Can you work these out from the model? Positions are in its coordinate system, mm. A direction names the side the tool comes from. Give positions to 0.01 mm unless a question says otherwise; leave off trailing zeros. Order: outer loops, then holes, each group sorted by start corner. A loop starts at its lowest first (then second) coordinate and runs counter-clockwise, first axis right, second up. Notation, with made-up numbers: M 87,68.5 L 137,68.5 A7 ccw 137,74.5 Z; hole C 83.25,56 d5. An arc over 180 degrees is marked long. Answer as a JSON object with one key per item and string values.
Autodesk Fusion 360 part; units mm, degrees
sketch "Sketch1" plane through (0, 0, 0) normal (0, 1, 0) x (1, 0, 0)
  line L0 (13.25, -10.25) -> (-13.25, -10.25)
  line L1 (-13.25, -10.25) -> (-13.25, 10.25)
  line L2 (-13.25, 10.25) -> (13.25, 10.25)
  line L3 (13.25, 10.25) -> (13.25, -10.25)
  line L4 (13.25, -10.25) -> (-13.25, 10.25) construction
  line L5 (-13.25, -10.25) -> (13.25, 10.25) construction
  line L6 (-13.25, 10.25) -> (-17.65, 10.25)
  line L7 (-17.65, 10.25) -> (-17.65, 0.25)
  line L8 (-17.65, 0.25) -> (-13.25, 0.25)
  dimension "d1" = 26.5
  dimension "d2" = 20.5
  dimension "d3" = 10
  dimension "d4" = 4.4
extrude "Extrude1" add sketch "Sketch1" along normal blind 1.85
sketch "Sketch2" plane through (0, 1.85, 0) normal (0, 1, 0) x (-1, 0, 0)
  line L0 (-13.25, -10.25) -> (17.65, -10.25)
  line L1 (17.65, -10.25) -> (17.65, -0.25)
  line L2 (17.65, -0.25) -> (13.25, -0.25)
  line L3 (13.25, -0.25) -> (13.25, 10.25)
  line L4 (13.25, 10.25) -> (-13.25, 10.25)
  line L5 (-13.25, 10.25) -> (-13.25, -10.25)
  line L6 (-11, -10.25) -> (-3.4, -10.25)
  line L7 (-3.4, -10.25) -> (-3.4, -5.55)
  line L8 (-3.4, -5.55) -> (-11, -5.55)
  line L9 (-11, -5.55) -> (-11, -10.25)
  dimension "d7" = 7.6
  dimension "d8" = 4.7
  dimension "d9" = 2.25
extrude "Extrude2" add sketch "Sketch2" along normal blind 3.2 contours L0 L6 L7 L8 L9
sketch "Sketch3" plane through (0, 0, 0) normal (0, -1, 0) x (1, 0, 0)
  line L0 (-17.65, -10.25) -> (13.25, -10.25)
  line L1 (13.25, -10.25) -> (13.25, 10.25)
  line L2 (13.25, 10.25) -> (-13.25, 10.25)
  line L3 (-13.25, 10.25) -> (-13.25, -0.25)
  line L4 (-13.25, -0.25) -> (-17.65, -0.25)
  line L5 (-17.65, -0.25) -> (-17.65, -10.25)
  line L6 (-10.5, 10.25) -> (10, 10.25)
  line L7 (10, 10.25) -> (10, -10.25)
  line L8 (10, -10.25) -> (-10.5, -10.25)
  line L9 (-10.5, -10.25) -> (-10.5, 10.25)
  dimension "d12" = 20.5
  dimension "d13" = 3.25
extrude "Extrude3" add sketch "Sketch3" along normal blind 3 contours L0 L2 L6 L7 L8 L9
sketch "Sketch4" plane through (-17.65, 0, 0) normal (-1, 0, 0) x (0, 0, 1)
  line L0 (-10.25, 0) -> (-0.25, 0)
  line L1 (-0.25, 0) -> (-0.25, 1.85)
  line L2 (-0.25, 1.85) -> (-10.25, 1.85)
  line L3 (-10.25, 1.85) -> (-10.25, 0)
  line L4 (-8.5, 3.05) -> (-2, 3.05)
  line L5 (-2, 3.05) -> (-2, -3.45)
  line L6 (-2, -3.45) -> (-8.5, -3.45)
  line L7 (-8.5, -3.45) -> (-8.5, 3.05)
  dimension "d16" = 6.5
  dimension "d17" = 6.5
  dimension "d18" = 1.2
  dimension "d19" = 1.75
extrude "Extrude4" add sketch "Sketch4" along normal blind 1.7 contours L0 L2 L5 L7 | L0 L5 L6 L7 | L2 L4 L5 L7
sketch "Sketch5" plane through (-19.35, 0, 0) normal (-1, 0, 0) x (0, 0, 1)
  line L0 (-8.5, -3.45) -> (-2, -3.45)
  line L1 (-2, -3.45) -> (-2, 3.05)
  line L2 (-2, 3.05) -> (-8.5, 3.05)
  line L3 (-8.5, 3.05) -> (-8.5, -3.45)
  circle A0 centre (-5.25, -0.2) radius 2.65
  line L4 (-5.25, -0.2) -> (-5.25, 3.05) construction
  line L5 (-5.25, -0.2) -> (-5.25, -3.45) construction
  dimension "d22" = 5.3
extrude "Extrude5" add sketch "Sketch5" along normal blind 2.85 contours A0
sketch "Sketch6" plane through (-22.2, 0, 0) normal (-1, 0, 0) x (0, 0, 1)
  circle A0 centre (-5.25, -0.2) radius 2.65
  circle A1 centre (-5.25, -0.2) radius 5
  dimension "d25" = 10
extrude "Extrude6" add sketch "Sketch6" along normal blind 20.75 contours A0 | A1
sketch "Sketch7" plane through (-42.95, 0, 0) normal (-1, 0, 0) x (0, 0, 1)
  circle A0 centre (-5.25, -0.2) radius 5
  line L0 (-3.5, -3.45) -> (-7, -3.45)
  line L1 (-7, -3.45) -> (-7, 3.05)
  line L2 (-7, 3.05) -> (-3.5, 3.05)
  line L3 (-3.5, 3.05) -> (-3.5, -3.45)
  line L4 (-3.5, -3.45) -> (-7, 3.05) construction
  line L5 (-7, -3.45) -> (-3.5, 3.05) construction
  point P0 (-5.25, -0.2)
  dimension "d28" = 6.5
  dimension "d29" = 3.5
extrude "Extrude7" add sketch "Sketch7" along normal blind 6.3 contours L0 L1 L2 L3
sketch "Sketch8" plane through (0, 3.05, 0) normal (0, 1, 0) x (-1, 0, 0)
  line L0 (42.95, -3.5) -> (42.95, -7)
  line L1 (42.95, -7) -> (49.25, -7)
  line L2 (49.25, -7) -> (49.25, -3.5)
  line L3 (49.25, -3.5) -> (42.95, -3.5)
  circle A0 centre (49.25, -5.25) radius 4.75
  dimension "d32" = 9.5
extrude "Extrude8" add sketch "Sketch8" along normal blind 80 contours L1 L2 L3 A0 | L1 L2 L3 A0
extrude "Extrude9" add 1 faces at (-50.8333, 3.05, -5.25) along direction (0, -1, 0) blind 4
fillet "Fillet1" radius 3 1 edges at (-44.8214, 83.05, -6.9677)
1) I want a section at B-B on x = -21. Write out the boundary of the cut face in (y, z).
Results found:
{"outline": "C -0.2,-5.25 d5.3"}
2) I want a section at A-A on z = 4. Write out the boundary of the cut face in (x, y), and give its area (3 significant figures).
Results found:
{"outline": "M -13.25,0 L -10.5,0 L -10.5,-3 L 10,-3 L 10,0 L 13.25,0 L 13.25,1.85 L -13.25,1.85 Z", "area": "111 mm²"}
3) For faces 4 (the face through (-45, -2, -7)), 5 (the face through (3.4, 3, -8)), 6 (the face through (7, 3, -5.55)), 7 (the face through (7, 5.05, -8)), 8 (the face through (-32.43, 4.236, -2.943)), which set-ups out of +Z, -Z, +X, -X, +Y, -Y let a thin tool reach every point of the face, with its end or its side?
Results found:
{"face 4": "-Z, -Y", "face 5": "+Z, -Z, +Y", "face 6": "+Z, +X, +Y", "face 7": "+Z, -Z, +X, +Y", "face 8": "none"}
4) I want a section at D-D on x = -7.5. Write out the boundary of the cut face in (y, z).
Results found:
{"outline": "M -3,-10.25 L 1.85,-10.25 L 1.85,10.25 L -3,10.25 Z"}
5) I need wall thicknesses on L1, parallel to Y at x = 10.5, z = -4; L2, parallel to X at y = -1, z = 8.5; L3, parallel to Y at x = -1, z = -4.25. Which ranges of each line are inside material? Lowest first, please.
Results found:
{"L1": "y = 0 to 1.85", "L2": "x = -10.5 to 10", "L3": "y = -3 to 1.85"}
6) I'm going to push flat-ended pins straight in: pin 1 Ø12 at (x, z) = (-46.5, 5.5) entering from -Y; pin 2 Ø5 at (x, z) = (6.5, -7) entering from +Y; pin 3 Ø0.9 at (y, z) = (1, -9.5) entering from -X; pin 4 Ø1.5 at (y, z) = (0.5, 3.5) entering from -X. Where does each tip first touch, or does it pass through?
Results found:
{"pin 1": "passes through", "pin 2": "stops at y = 5.05", "pin 3": "stops at x = -52.1", "pin 4": "stops at x = -13.25"}
7) Thinking about a two-plate mould opening in X: for faces 1 (the face through (11, 3, -8)), 2 (the face through (-18, -3.45, -5)), 3 (the face through (-18, 0, -2)), which applies, pulls with the +X half, pulls with the -X half, needs draft (parallel to the pull), parting line crosses it, or undercut?
Results found:
{"face 1": "pulls with the +X half", "face 2": "needs draft", "face 3": "undercut"}
8) I want a section at C-C on y = 72.5. Write out the boundary of the cut face in (x, z), and give its area (3 significant figures).
Results found:
{"outline": "C -49.25,-5.25 d9.5", "area": "70.9 mm²"}
